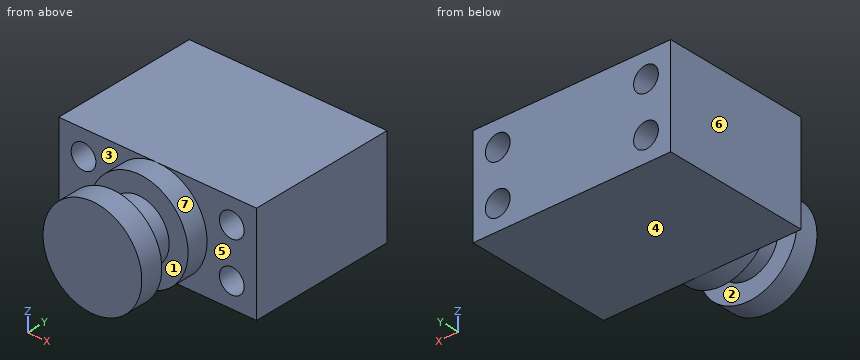
from build123d import *

# Parameters (mm, degrees)
F0_W     = 101.6
F0_H     = 50.8
F1_DEPTH = 76.2
F2_R     = 6.35
F3_DEPTH = 76.201
F4_W     = 25.4
F4_H     = 38.1
F6_W     = 0.105277
F6_H     = 15.308836
F6_W_2   = 9.73333


with BuildPart() as f1:
    # F0 (on Front) → F1 (new body)
    with BuildSketch(Plane.XZ):
        Rectangle(F0_W, F0_H)
    extrude(amount=F1_DEPTH)

    # F2 (on face) → F3 (cut, through all)
    with BuildSketch(Plane.XZ.offset(76.2)):
        with Locations((-38.1, 12.7)):
            Circle(F2_R)
        with Locations((-38.1, -12.7)):
            Circle(F2_R)
        with Locations((38.1, 12.7)):
            Circle(F2_R)
        with Locations((38.1, -12.7)):
            Circle(F2_R)
    extrude(amount=-F3_DEPTH, mode=Mode.SUBTRACT)

    # F4 (on Top) → F5 (revolve)
    with BuildSketch(Plane.XY):
        with Locations((-12.7, -95.25)):
            Rectangle(F4_W, F4_H)
    revolve(axis=Axis((0, -95.25, 0), (0, -1, 0)))

    # F6 (on Top) → F7 (revolve, cut)
    with BuildSketch(Plane.XY):
        with Locations((-25.452638, -94.963487)):
            Rectangle(F6_W, F6_H)
        with Locations((-20.533335, -94.963487)):
            Rectangle(F6_W_2, F6_H)
    revolve(axis=Axis((0, -61.931949, 0), (0, 1, 0)), mode=Mode.SUBTRACT)


solid = f1.part
Geometry: final body of the model. Coordinates: model frame, mm. Face numbers are marked on the shaded views. A direction names the side the tool comes from. Coordinates: 2 decimals unless noted, no trailing zeros. Loops run counter-clockwise (first coordinate to the right, second up) from the corner with the lowest first, then second, coordinate; pieces in that order, holes last. Notation, with made-up numbers: (82, 32) - (120, 32) arc R16 cw to (120, 42) - close; hole circle Ø8 at (73.5, 81). An arc over 180 degrees is marked (long way). Put each result on its own line as item: value. Start each with the question number.
Q1. Cut plane D-D, the plane z = 0. Return loops of the section in (x, y), and give its area (3 significant figures).
Q2. Pull-direction query (Y, two-part tool) for the marked faces 1, 2, 3 and 4; classes: released by +Y, released by -Y, zero draft, split by the parting line, or undercut.
Q3. Cut plane A-A, the plane x = -38.1. Return loops of the section in (y, z).
Q4. Pin query (flat end, axial travel): pin 1 Ø14.5 at (x, z) = (-38.1, 12.7) entering from -Y; pin 2 Ø1 at (y, z) = (-93, 12) entering from +X. Return the tip coordinate at first contact, or that it passes through.
Q5. Cut plane C-C, the plane x = 20.5. Return loops of the section in (y, z).
Q6. Set-up query: the marked faces 5, 6 and 7. Return all of +Z, -Z, +X, -X, +Y, -Y with unobstructed straight access to the full face (end or side cutting, diameter ignored); none if empty.
Q7. Cut plane B-B, the plane y = -9. Return loops of the section in (x, z).
Q8. Line query: line 1 (Z direction, x = 38.1, y = -48); line 2 (X direction, y = -35, z = 12); line 3 (Y direction, x = -18.5, z = -8). Output: solid intervals per line, ascending.
Filled sheet:
1. outline: (-50.8, -76.2) - (-25.4, -76.2) - (-25.4, -87.31) - (-15.67, -87.31) - (-15.67, -102.62) - (-25.4, -102.62) - (-25.4, -114.3) - (25.4, -114.3) - (25.4, -102.62) - (15.67, -102.62) - (15.67, -87.31) - (25.4, -87.31) - (25.4, -76.2) - (50.8, -76.2) - (50.8, 0) - (-50.8, 0) - close
1. area: 9,380 mm²
2. face 1: undercut
2. face 2: undercut
2. face 3: released by -Y
2. face 4: zero draft
3. outline: (-76.2, -25.4) - (0, -25.4) - (0, -19.05) - (-76.2, -19.05) - close; (-76.2, -6.35) - (0, -6.35) - (0, 6.35) - (-76.2, 6.35) - close; (-76.2, 19.05) - (0, 19.05) - (0, 25.4) - (-76.2, 25.4) - close
4. pin 1: y = -76.2
4. pin 2: x = 10.64
5. outline: (-114.3, -15) - (-102.62, -15) - (-102.62, 15) - (-114.3, 15) - close; (-87.31, -15) - (-76.2, -15) - (-76.2, -25.4) - (0, -25.4) - (0, 25.4) - (-76.2, 25.4) - (-76.2, 15) - (-87.31, 15) - close
6. face 5: +X, -Y
6. face 6: +Z, -Z, -X, +Y, -Y
6. face 7: -Y
7. outline: (-50.8, -25.4) - (50.8, -25.4) - (50.8, 25.4) - (-50.8, 25.4) - close; hole circle Ø12.7 at (-38.1, -12.7); hole circle Ø12.7 at (-38.1, 12.7); hole circle Ø12.7 at (38.1, -12.7); hole circle Ø12.7 at (38.1, 12.7)
8. line 1: -25.4 to -19.05, -6.35 to 6.35, 19.05 to 25.4
8. line 2: -50.8 to -44.41, -31.79 to 31.79, 44.41 to 50.8
8. line 3: -114.3 to -102.62, -87.31 to 0
